```python
from build123d import *

# Parameters (mm, degrees)
SKETCH_2_W          = 43
SKETCH_2_H          = 40.2
SKETCH_2_R          = 1.75
EXTRUDE_1_DEPTH     = 10
EXTRUDE_1_2_DEPTH   = 10
SKETCH_3_W          = 43
SKETCH_3_H          = 36.5
EXTRUDE_2_DEPTH     = 10
SKETCH_4_W          = 121.9
SKETCH_4_H          = 150
EXTRUDE_3_DEPTH     = 10
SKETCH_6_W          = 121.9
SKETCH_6_H          = 36.5
EXTRUDE_4_DEPTH     = 10
EXTRUDE_5_REACH     = 285.745
SKETCH_7_R          = 5
FILLET_1_R          = 5
FILLET_2_R          = 5
EXTRUDE_6_DEPTH     = 10
SKETCH_9_W          = 79
SKETCH_9_H          = 27
CUT_EXTRUDE_1_DEPTH = 3
SKETCH_10_W         = 79
SKETCH_10_H         = 13
CUT_EXTRUDE_2_DEPTH = 293.327316548
RIB_16_REACH        = 320.066
SKETCH_11_WALL_W    = 685.378322466
SKETCH_11_WALL_H    = 5
SKETCH_12_W         = 10
SKETCH_12_H         = 130
EXTRUDE_7_DEPTH     = 42.5
SKETCH_13_R         = 2
CUT_EXTRUDE_3_DEPTH = 42.5
SKETCH_14_R         = 2.5
EXTRUDE_8_DEPTH     = 70
SKETCH_15_W         = 70
SKETCH_15_H         = 80
CUT_EXTRUDE_4_DEPTH = 60
RIB_17_REACH        = 321.176
SKETCH_16_WALL_W    = 687.174412562
SKETCH_16_WALL_H    = 5
FILLET_4_R          = 5
FILLET_5_R          = 5
FILLET_6_R          = 5
SKETCH_17_R         = 2.5
CUT_EXTRUDE_5_DEPTH = 293.947371553


with BuildPart() as part:
    # Sketch 2 → Extrude 1 (new body)
    with BuildSketch(Plane.XY):
        with Locations((-39.45, -100)):
            Rectangle(SKETCH_2_W, SKETCH_2_H)
        with Locations((-50.2, -85)):
            Circle(SKETCH_2_R, mode=Mode.SUBTRACT)
        with Locations((-26, -85)):
            Circle(SKETCH_2_R, mode=Mode.SUBTRACT)
        with Locations((-50.2, -115)):
            Circle(SKETCH_2_R, mode=Mode.SUBTRACT)
        with Locations((-26, -115)):
            Circle(SKETCH_2_R, mode=Mode.SUBTRACT)
    extrude(amount=EXTRUDE_1_DEPTH)



with BuildPart() as body_2:
    # Sketch 2 → Extrude 1 2 (new body)
    with BuildSketch(Plane.XY):
        with Locations((39.45, -100)):
            Rectangle(SKETCH_2_W, SKETCH_2_H)
        with Locations((50.2, -85)):
            Circle(SKETCH_2_R, mode=Mode.SUBTRACT)
        with Locations((26, -85)):
            Circle(SKETCH_2_R, mode=Mode.SUBTRACT)
        with Locations((26, -115)):
            Circle(SKETCH_2_R, mode=Mode.SUBTRACT)
        with Locations((50.2, -115)):
            Circle(SKETCH_2_R, mode=Mode.SUBTRACT)
    extrude(amount=EXTRUDE_1_2_DEPTH)


with BuildPart() as part_1:
    add(part.part)

    add(body_2.part)  # Extrude 2 merges body 2
    # Sketch 3 → Extrude 2 (add)
    with BuildSketch(Plane.XZ.offset(120.1)):
        with Locations((39.45, -8.25)):
            Rectangle(SKETCH_3_W, SKETCH_3_H)
        with Locations((-39.45, -8.25)):
            Rectangle(SKETCH_3_W, SKETCH_3_H)
    extrude(amount=EXTRUDE_2_DEPTH)

    # Sketch 4 → Extrude 3 (add)
    with BuildSketch(Plane(origin=(0, 0, -26.5), x_dir=(-1, 0, 0), z_dir=(0, 0, -1))):
        with Locations((0, -195.1)):
            Rectangle(SKETCH_4_W, SKETCH_4_H)
    extrude(amount=EXTRUDE_3_DEPTH)

    # Sketch 6 → Extrude 4 (add)
    with BuildSketch(Plane(origin=(0, -79.9, 0), x_dir=(1, 0, 0), z_dir=(0, 1, 0))):
        with Locations((0, 8.25)):
            Rectangle(SKETCH_6_W, SKETCH_6_H)
    extrude(amount=EXTRUDE_4_DEPTH)

    # Sketch 7 → Extrude 5 (add, up to next)
    with BuildSketch(Plane.ZY.offset(-17.95), mode=Mode.PRIVATE) as extrude_5_sk1:
        with Locations(Location((5, -125.1, 0), (0, 0, 270))):
            Circle(SKETCH_7_R)
    extrude_5_tool1 = extrude(extrude_5_sk1.sketch, amount=EXTRUDE_5_REACH, mode=Mode.PRIVATE) - part_1.part
    add(extrude_5_tool1.solids().sort_by_distance((17.95, -125.1, 5))[0])

    # Fillet 1
    fillet_1_edges = [part_1.edges().sort_by_distance(p)[0] for p in [
        (-39.45, -130.1, 10),
        (39.45, -130.1, 10),
    ]]
    fillet(fillet_1_edges, radius=FILLET_1_R - 0.0001)  # a hair under: the kernel refuses the full size

    # Fillet 2
    fillet_2_edges = [part_1.edges().sort_by_distance(p)[0] for p in [
        (-39.45, -130.1, -26.5),
        (39.45, -130.1, -26.5),
    ]]
    fillet(fillet_2_edges, radius=FILLET_2_R)

    # Sketch 8 → Extrude 6 (add)
    with BuildSketch(Plane(origin=(0, 0, -26.5), x_dir=(-1, 0, 0), z_dir=(0, 0, -1))):
        Polygon((-60.95, -79.9), (60.95, -79.9), (60.95, -59.9), (103, -59.9), (103, -39.9), (-103, -39.9), (-103, -59.9), (-60.95, -59.9), align=None)
    extrude(amount=EXTRUDE_6_DEPTH)

    # Sketch 9 → Cut-Extrude 1 (cut)
    with BuildSketch(Plane(origin=(0, 0, -36.5), x_dir=(-1, 0, 0), z_dir=(0, 0, -1))):
        with Locations((0, -53.4)):
            Rectangle(SKETCH_9_W, SKETCH_9_H)
    extrude(amount=-CUT_EXTRUDE_1_DEPTH, mode=Mode.SUBTRACT)

    # Sketch 10 → Cut-Extrude 2 (cut, through all)
    with BuildSketch(Plane(origin=(0, 0, -33.5), x_dir=(-1, 0, 0), z_dir=(0, 0, -1))):
        with Locations((0, -60.4)):
            Rectangle(SKETCH_10_W, SKETCH_10_H)
    extrude(amount=-CUT_EXTRUDE_2_DEPTH, mode=Mode.SUBTRACT)

    # Sketch 11 wall → Rib 16 (add, up to next)
    with BuildSketch(Plane(origin=(-60.95, -54.9, -8.25), x_dir=(0, 0.634965075677, -0.772540842073), z_dir=(0, -0.772540842073, -0.634965075677)), mode=Mode.PRIVATE) as rib_16_sk1:
        with Locations((0, 2.5)):
            Rectangle(SKETCH_11_WALL_W, SKETCH_11_WALL_H)
    rib_16_tool1 = extrude(rib_16_sk1.sketch, amount=RIB_16_REACH, mode=Mode.PRIVATE) - part_1.part
    rib_16 = rib_16_tool1.solids().sort_by_distance((-60.95, -54.9, -8.25))[0]
    add(rib_16)

    # Mirror 1: Rib 16 across plane
    add(rib_16.mirror(Plane(origin=(0, 0, 0), x_dir=(0, 0, 1), z_dir=(1, 0, 0))))

    # Sketch 12 → Extrude 7 (add)
    with BuildSketch(Plane.ZY.offset(60.95)):
        with Locations((-31.5, -205.1)):
            Rectangle(SKETCH_12_W, SKETCH_12_H)
    extrude_7 = extrude(amount=EXTRUDE_7_DEPTH)

    # Mirror 2: Extrude 7 across plane
    add(extrude_7.mirror(Plane(origin=(0, 0, 0), x_dir=(0, 0, 1), z_dir=(1, 0, 0))))

    # Sketch 13 → Cut-Extrude 3 (cut)
    with BuildSketch(Plane.XY.offset(-26.5)):
        with Locations((98.45, -265.1)):
            Circle(SKETCH_13_R)
        with Locations((98.45, -241.1)):
            Circle(SKETCH_13_R)
        with Locations((69.95, -265.1)):
            Circle(SKETCH_13_R)
        with Locations((69.95, -241.1)):
            Circle(SKETCH_13_R)
    cut_extrude_3 = extrude(amount=-CUT_EXTRUDE_3_DEPTH, mode=Mode.SUBTRACT)

    # Mirror 3: Cut-Extrude 3 across plane
    add(cut_extrude_3.mirror(Plane(origin=(0, 0, 0), x_dir=(0, 0, 1), z_dir=(1, 0, 0))), mode=Mode.SUBTRACT)

    # Sketch 14 → Extrude 8 (add)
    with BuildSketch(Plane.XY.offset(-26.5)):
        with Locations(Location((-45, -260.1, 0), (0, 0, 180))):
            Circle(SKETCH_14_R)
        with Locations(Location((45, -260.1, 0), (0, 0, 180))):
            Circle(SKETCH_14_R)
        with Locations(Location((-45, -190.1, 0), (0, 0, 180))):
            Circle(SKETCH_14_R)
        with Locations(Location((45, -190.1, 0), (0, 0, 180))):
            Circle(SKETCH_14_R)
    extrude(amount=EXTRUDE_8_DEPTH)

    # Sketch 15 → Cut-Extrude 4 (cut)
    with BuildSketch(Plane.XY.offset(-26.5)):
        with Locations((0, -230.1)):
            Rectangle(SKETCH_15_W, SKETCH_15_H)
    extrude(amount=-CUT_EXTRUDE_4_DEPTH, mode=Mode.SUBTRACT)

    # Sketch 16 wall → Rib 17 (add, up to next)
    with BuildSketch(Plane(origin=(-60.95, -144.460273185, -9.079855192), x_dir=(0, -0.668057923191, -0.744109273737), z_dir=(0, -0.744109273737, 0.668057923191)), mode=Mode.PRIVATE) as rib_17_sk1:
        with Locations((0, 2.5)):
            Rectangle(SKETCH_16_WALL_W, SKETCH_16_WALL_H)
    rib_17_tool1 = extrude(rib_17_sk1.sketch, amount=-RIB_17_REACH, mode=Mode.PRIVATE) - part_1.part
    rib_17 = rib_17_tool1.solids().sort_by_distance((-60.95, -144.460273185, -9.079855192))[0]
    add(rib_17)

    # Mirror 4: Rib 17 across plane
    add(rib_17.mirror(Plane(origin=(0, 0, 0), x_dir=(0, 0, 1), z_dir=(1, 0, 0))))

    # Fillet 4
    fillet_4_edges = [part_1.edges().sort_by_distance(p)[0] for p in [
        (-103, -39.9, -31.5),
        (103, -39.9, -31.5),
    ]]
    fillet(fillet_4_edges, radius=FILLET_4_R)

    # Fillet 5
    fillet_5_edges = [part_1.edges().sort_by_distance(p)[0] for p in [
        (-103.45, -270.1, -31.5),
        (103.45, -270.1, -31.5),
    ]]
    fillet(fillet_5_edges, radius=FILLET_5_R)

    # Fillet 6
    fillet_6_edges = [part_1.edges().sort_by_distance(p)[0] for p in [
        (-35, -190.1, -31.5),
        (35, -190.1, -31.5),
        (-35, -230.1, -26.5),
        (35, -230.1, -26.5),
        (0, -190.1, -26.5),
    ]]
    fillet(fillet_6_edges, radius=FILLET_6_R)

    # Sketch 17 → Cut-Extrude 5 (cut, through all)
    with BuildSketch(Plane.XY.offset(10)):
        with Locations((38.5, -90.6)):
            Circle(SKETCH_17_R)
        with Locations((-38.5, -90.6)):
            Circle(SKETCH_17_R)
    extrude(amount=-CUT_EXTRUDE_5_DEPTH, mode=Mode.SUBTRACT)


solid = part_1.part
```
Build history of the part. All positions in model axes, mm. A direction names the side the tool comes from. Round coordinates to 2 decimals unless told otherwise and drop trailing zeros. Order: outer loops, then holes, each group sorted by start corner. A loop starts at its lowest first (then second) coordinate and runs counter-clockwise, first axis right, second up. Notation, with made-up numbers: (24, 43) -> (34, 43) arc R15 ccw to (34, 68) -> close; hole circle Ø11 at (-7.5, -27). An arc over 180 degrees is marked (long way). Answer in a Markdown table with one row per item.
1) Band-saw the part on B-B on y = -223.5. Give the cut face in (x, z).
Values:
| item | result |
|---|---|
| outline | (-103.45, -36.5) -> (-35, -36.5) -> (-35, -31.5) arc R5 ccw to (-40, -26.5) -> (-103.45, -26.5) -> close; (35, -36.5) -> (103.45, -36.5) -> (103.45, -26.5) -> (40, -26.5) arc R5 ccw to (35, -31.5) -> close |
2) Band-saw the part on D-D on z = 37.5. Give the cut face in (x, y).
Values:
| item | result |
|---|---|
| outline | circle Ø5 at (-45, -260.1); circle Ø5 at (-45, -190.1); circle Ø5 at (45, -260.1); circle Ø5 at (45, -190.1) |
3) Band-saw the part on C-C on x = 3. Give the cut face in (y, z), and give its area (3 significant figures).
Values:
| item | result |
|---|---|
| outline | (-190.1, -36.5) -> (-120.1, -36.5) -> (-120.1, -26.5) -> (-185.1, -26.5) arc R5 ccw to (-190.1, -31.5) -> close; circle Ø10 at (-125.1, 5); (-79.9, -36.5) -> (-66.9, -36.5) -> (-66.9, -26.5) -> (-69.9, -26.5) -> (-69.9, 10) -> (-79.9, 10) -> close; (-53.9, -33.5) -> (-39.9, -33.5) -> (-39.9, -26.5) -> (-53.9, -26.5) -> close |
| area | 1,370 mm2 |
4) Pin check, flat tips, straight feed: P1, Ø5.5, axis at x = 26, y = -85, coming from the -Z side; P2, Ø23, axis at y = -89.5, z = -15, coming from the +X side; P3, Ø8, axis at x = 7.5, z = 7.5, coming from the +Y side. Stop position of each tip, or through.
Values:
| item | result |
|---|---|
| P1 | z = 0 |
| P2 | x = 60.95 |
| P3 | y = -69.9 |
5) Which spindle directions (+Z, -Z, +X, -X, +Y, -Y) get a long thin tool onto all of the face, cutting with end or side? Do faces 1 (the flat face through (-1, -69.9, -9)), 2 (the cylindrical face through (43.85, -257.88, 8.01)), 3 (the flat face through (55.95, -142, -18)), 4 (the flat face through (1, -120.1, -30)), 5 (the flat face through (-82, -140.1, -32)). Say none if no direction does.
Values:
| item | result |
|---|---|
| face 1 | +Z, +Y |
| face 2 | +Z |
| face 3 | +Z, -Y |
| face 4 | -Z, +X, -X |
| face 5 | +Z, -Z, -X |
6) Mould opens along Y. For faces 6 (the flat face through (82, -59.9, -31)), 7 (the cylindrical face through (101.5, -41.33, -31.57)), 8 (the cylindrical face through (-101.95, -268.67, -31.43)) say: released by +Y, released by -Y, zero draft, split by the parting line, or undercut.
Values:
| item | result |
|---|---|
| face 6 | undercut |
| face 7 | released by +Y |
| face 8 | released by -Y |
7) Wall check: L1, parallel to X at y = -241, z = -32; L2, parallel to X at y = -85, z = 3; L3, parallel to Y at x = -69.95, z = -29. Give the ranges that are in metal, low to high.
Values:
| item | result |
|---|---|
| L1 | -103.45 to -100.45, -96.45 to -71.95, -67.95 to -35, 35 to 67.95, 71.95 to 96.45, 100.45 to 103.45 |
| L2 | -60.95 to -51.95, -48.45 to -27.75, -24.25 to -17.95, 17.95 to 24.25, 27.75 to 48.45, 51.95 to 60.95 |
| L3 | -270.1 to -267.1, -263.1 to -243.1, -239.1 to -140.1, -59.9 to -39.9 |
8) Band-saw the part on A-A on x = -78. Give the cut face in (y, z), and give its area (3 significant figures).
Values:
| item | result |
|---|---|
| outline | (-270.1, -36.5) -> (-140.1, -36.5) -> (-140.1, -26.5) -> (-270.1, -26.5) -> close; (-59.9, -36.5) -> (-39.9, -36.5) -> (-39.9, -26.5) -> (-59.9, -26.5) -> close |
| area | 1,500 mm2 |
